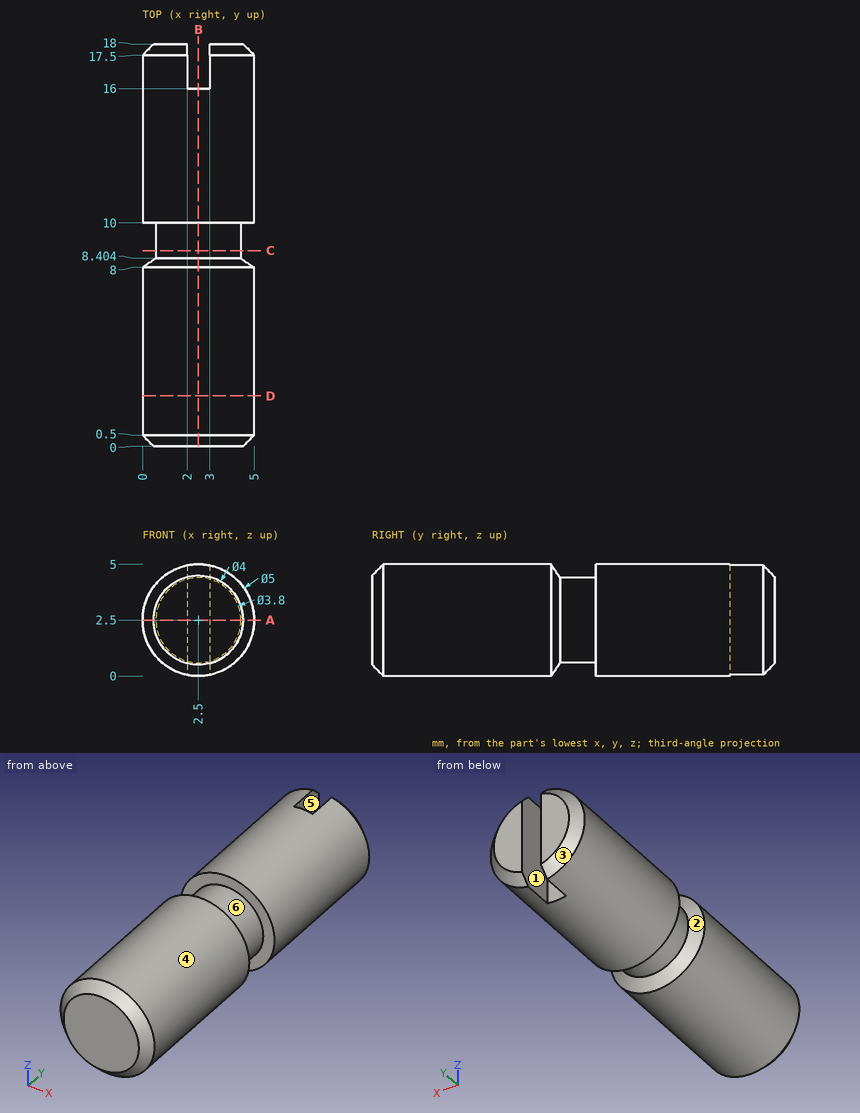
The drawing under review shows one solid part. Ordinate dimensions are in mm from its lowest x, y, z. A direction names the side the tool comes from. Coordinates: 2 decimals unless noted, no trailing zeros. Order: outer loops, then holes, each group sorted by start corner. A loop starts at its lowest first (then second) coordinate and runs counter-clockwise, first axis right, second up. Notation, with made-up numbers: (50, -37) -> (87, -37) arc R5 ccw to (87, -28) -> close; hole circle Ø8 at (-27.5, 77). An arc over 180 degrees is marked (long way). Answer in a Markdown table with one row per item. Add a question column.
Item 1: Machinability: for the marked faces 4, 5 and 6, which of the approach directions +Z, -Z, +X, -X, +Y, -Y give a long, thin tool a straight path to every point of the face, cutting with its end or side? Answer none if there is none.
Item 2: Clearance check with flat-ended pins moving along their axes: pin 1 (0.5 mm diameter, centred on x = 2.5, z = 2, fed in from +Y); pin 2 (2 mm diameter, centred on x = 4.5, y = 5, fed in from -Z); pin 3 (1 mm diameter, centred on y = 4, z = 1.5, fed in from +X). State where each tip first meets the part, or that it passes through.
Item 3: We need section D-D on y = 2.25. Write out the cut boundary in (x, z).
Item 4: We need section A-A on z = 2.5. Write out the cut boundary in (x, y) (1 decimal).
Item 5: Mouldability with a two-part tool opening along X and no side actions: class the marked faces 1, 2 and 3 as +X half, -X half, draft (parallel to the pull), parting line (faces both ways), or undercut.
Item 6: We need section C-C on y = 8.75. Write out the cut boundary in (x, z).
Item 7: To check wall thickness, follow probe 1 along Z at (x, y) = (4, 7.25); probe 2 along X at (y, z) = (17.25, 4.45) (1 decimal); probe 3 along Y at (x, z) = (1.55, 4.65). State the ranges of each line that lie inside material, in increasing order.
Item 8: We need section B-B on x = 2.5. Write out the cut boundary in (y, z) (1 decimal).
Final values:
| question | item | result |
|---|---|---|
| 1 | face 4 | +Y, -Y |
| 1 | face 5 | +Z, -Z, +Y |
| 1 | face 6 | none |
| 2 | pin 1 | stops at y = 16 |
| 2 | pin 2 | stops at z = 0.21 |
| 2 | pin 3 | stops at x = 4.95 |
| 3 | outline | circle Ø5 at (2.5, 2.5) |
| 4 | outline | (0, 0.5) -> (0.5, 0) -> (4.5, 0) -> (5, 0.5) -> (5, 8) -> (4.4, 8.4) -> (4.4, 10) -> (5, 10) -> (5, 17.5) -> (4.5, 18) -> (3, 18) -> (3, 16) -> (2, 16) -> (2, 18) -> (0.5, 18) -> (0, 17.5) -> (0, 10) -> (0.6, 10) -> (0.6, 8.4) -> (0, 8) -> close |
| 5 | face 1 | undercut |
| 5 | face 2 | parting line |
| 5 | face 3 | -X half |
| 6 | outline | circle Ø3.8 at (2.5, 2.5) |
| 7 | probe 1 | z = 0.5 to 4.5 |
| 7 | probe 2 | x = 0.9 to 2, 3 to 4.1 |
| 7 | probe 3 | y = 0.35 to 8.1, 10 to 17.65 |
| 8 | outline | (0, 0.5) -> (0.5, 0) -> (8, 0) -> (8.4, 0.6) -> (10, 0.6) -> (10, 0) -> (16, 0) -> (16, 5) -> (10, 5) -> (10, 4.4) -> (8.4, 4.4) -> (8, 5) -> (0.5, 5) -> (0, 4.5) -> close |
